from build123d import *

# Parameters (mm, degrees)
RESSALTO_EXTRUS_O1_DEPTH = 10
ESBO_O3_R                = 2
CORTE_EXTRUS_O1_DEPTH    = 15
CHANFRO1_SIZE            = 1.6
FILETE1_R                = 0.5
CHANFRO5_SIZE            = 2
ESBO_O4_R                = 2.5
CORTE_EXTRUS_O2_DEPTH    = 10
CHANFRO8_SIZE            = 1
FILETE2_R                = 0.5


with BuildPart() as part:
    # Esboço1 → Ressalto-extrusão1 (new body)
    with BuildSketch(Plane.XY):
        Polygon((1.886382163, -7.75), (-4.113617837, -7.75), (-4.113617837, -22.95), (15.886382163, -22.95), (15.886382163, -27.95), (-9.113617837, -27.95), (-9.113617837, 19.25), (37.886382163, 19.25), (37.886382163, 29.25), (42.886382163, 29.25), (42.886382163, 14.25), (-4.113617837, 14.25), (-4.113617837, -2.75), (1.886382163, -2.75), align=None)
    extrude(amount=RESSALTO_EXTRUS_O1_DEPTH)

    # Esboço3 → Corte-extrusão1 (cut)
    with BuildSketch(Plane.XZ.offset(27.95)):
        with Locations(Location((7.886382163, 5, 0), (0, 0, 270))):
            Circle(ESBO_O3_R)
    extrude(amount=-CORTE_EXTRUS_O1_DEPTH, mode=Mode.SUBTRACT)

    # Chanfro1
    chanfro1_edges = [part.edges().sort_by_distance(p)[0] for p in [
        (7.886382163, -27.95, 7),
    ]]
    chamfer(chanfro1_edges, length=CHANFRO1_SIZE)

    # Filete1
    filete1_edges = [part.edges().sort_by_distance(p)[0] for p in [
        (7.886382163, -22.95, 7),
    ]]
    fillet(filete1_edges, radius=FILETE1_R)

    # Chanfro5
    chanfro5_edges = [part.edges().sort_by_distance(p)[0] for p in [
        (15.886382163, -27.95, 5),
        (-9.113617837, -27.95, 5),
        (-9.113617837, 19.25, 5),
        (42.886382163, 14.25, 5),
        (-4.113617837, 14.25, 5),
        (1.886382163, -2.75, 5),
    ]]
    chamfer(chanfro5_edges, length=CHANFRO5_SIZE)

    # Esboço4 → Corte-extrusão2 (cut)
    with BuildSketch(Plane.ZY.offset(-37.886382163)):
        with Locations((5, 24.25)):
            Circle(ESBO_O4_R)
    extrude(amount=-CORTE_EXTRUS_O2_DEPTH, mode=Mode.SUBTRACT)

    # Chanfro8
    chanfro8_edges = [part.edges().sort_by_distance(p)[0] for p in [
        (-4.113617837, 4.75, 10),
        (15.386382163, 19.25, 0),
        (37.886382163, 24.25, 0),
        (40.386382163, 29.25, 0),
        (-4.113617837, 4.75, 0),
        (1.886382163, -6.25, 0),
        (37.886382163, 19.25, 5),
        (37.886382163, 29.25, 5),
        (42.886382163, 29.25, 5),
        (40.386382163, 29.25, 10),
        (37.886382163, 24.25, 10),
        (15.386382163, 19.25, 10),
        (1.886382163, -6.25, 10),
        (-9.113617837, -4.35, 0),
        (-9.113617837, -4.35, 10),
        (15.886382163, -24.45, 0),
        (3.386382163, -27.95, 0),
        (42.886382163, 22.75, 0),
        (19.386382163, 14.25, 0),
        (-2.113617837, -2.75, 0),
        (0.886382163, -3.75, 0),
        (14.886382163, -26.95, 0),
        (-8.113617837, -26.95, 0),
        (41.886382163, 15.25, 0),
        (-8.113617837, 18.25, 0),
        (-2.113617837, -2.75, 10),
        (19.386382163, 14.25, 10),
        (42.886382163, 22.75, 10),
        (3.386382163, -27.95, 10),
        (15.886382163, -24.45, 10),
        (0.886382163, -3.75, 10),
        (14.886382163, -26.95, 10),
        (-8.113617837, -26.95, 10),
        (41.886382163, 15.25, 10),
        (-8.113617837, 18.25, 10),
        (-3.113617837, 13.25, 0),
        (-3.113617837, 13.25, 10),
    ]]
    chamfer(chanfro8_edges, length=CHANFRO8_SIZE)

    # Filete2
    filete2_edges = [part.edges().sort_by_distance(p)[0] for p in [
        (42.886382163, 24.25, 2.5),
        (37.886382163, 24.25, 2.5),
    ]]
    fillet(filete2_edges, radius=FILETE2_R)


solid = part.part
Check sheet for the modelled part. Datum: model origin and axes. Units: mm. A direction names the side the tool comes from. Round coordinates to 2 decimals unless told otherwise and drop trailing zeros. Loops run counter-clockwise (first coordinate to the right, second up) from the corner with the lowest first, then second, coordinate; pieces in that order, holes last. Notation, with made-up numbers: M -2.5,19 L 51.5,19 A18 cw 51.5,34 Z; hole C 74,47 d5. An arc over 180 degrees is marked long. One line per item, written item: value.
(1) Access from +Z, -Z, +X, -X, +Y, -Y to the whole of each face (thin tool, end or side, straight path). Record for faces 4 (the face through (15.886, -24, 5)), 5 (the face through (15, 19.25, 5)), 6 (the face through (-2, -2.75, 5)), 7 (the face through (14.514, -26.605, 9.507)).
Computed values:
face 4: +Z, -Z, +X, -Y
face 5: +Z, -Z, -X, +Y
face 6: +Z, -Z, +X
face 7: +Z, +X, -Y
(2) Depth check by flat-ended pin: pin 1 Ø4 at (x, z) = (15, 3.5) entering from +Y; pin 2 Ø4 at (y, z) = (24, 4) entering from -X; pin 3 Ø3.5 at (y, z) = (-6, 4) entering from +X. Enter the tip coordinate at first touch or a pass-through.
Computed values:
pin 1: stops at y = 19.25
pin 2: stops at x = 37.89
pin 3: stops at x = 1.89
(3) Sectioned sample at A-A, the plane y = 24.25. Record the cut outline in (x, z), then the cut area to 3 significant figures.
Computed values:
outline: M 37.89,1 L 38.89,0 L 41.89,0 L 42.89,1 L 42.89,2 A0.5 ccw 42.39,2.5 L 38.39,2.5 A0.5 ccw 37.89,2 Z; M 37.89,8 A0.5 ccw 38.39,7.5 L 42.39,7.5 A0.5 ccw 42.89,8 L 42.89,9 L 41.89,10 L 38.89,10 L 37.89,9 Z
area: 22.8 mm^2
(4) Thickness scan on line 1 (Y direction, x = 40.8, z = 5); line 2 (Y direction, x = 2, z = 5.5); line 3 (X direction, y = -25.3, z = 5). Record the ranges inside material, lowest first.
Computed values:
line 1: y = 14.25 to 21.75, 26.75 to 29.25
line 2: y = -27.95 to -22.95, 14.25 to 19.25
line 3: x = -9.11 to 5.89, 9.89 to 15.89
(5) Release check for a two-part mould opening along Z. For faces 1 (the face through (0.52, -4.08, 0.51)), 2 (the face through (0.52, -4.08, 9.49)), 3 (the face through (40.36, 26.36, 6.34)) record: +Z half, -Z half, draft (parallel to the pull), parting line (faces both ways), or undercut.
Computed values:
face 1: -Z half
face 2: +Z half
face 3: undercut
(6) Sectioned sample at B-B, the plane y = 8.5. Record the cut outline in (x, z).
Computed values:
outline: M -9.11,1 L -8.11,0 L -5.11,0 L -4.11,1 L -4.11,9 L -5.11,10 L -8.11,10 L -9.11,9 Z
(7) Sectioned sample at C-C, the plane z = 5. Count the separate pieces of the cut face and the enclosed holes in it, then the cut area to 3 significant figures.
Computed values:
separate pieces: 3
enclosed holes: 0
area: 595 mm^2
